```python
from build123d import *

# Parameters (mm, degrees)
F1_DEPTH = 9
F2_DEPTH = 2


with BuildPart() as f1:
    # F0 (on Top) → F1 (new body)
    with BuildSketch(Plane.XY):
        with BuildLine():
            ThreePointArc((3.4640958416, -2), (3.863698102, -1.0352762805), (3.999995, 0))
            ThreePointArc((3.999995, 0), (3.863698102, 1.0352762805), (3.4640958416, 2))
            Line((3.4640958416, 2), (-3.4640958416, 2))
            ThreePointArc((-3.4640958416, 2), (-3.999995, 0), (-3.4640958416, -2))
            Line((-3.4640958416, -2), (3.4640958416, -2))
        make_face()
        with BuildLine():
            Line((-3.4640958416, 2), (3.4640958416, 2))
            ThreePointArc((3.4640958416, 2), (0, 3.999995), (-3.4640958416, 2))
        make_face()
        with BuildLine():
            ThreePointArc((-3.4640958416, -2), (0, -3.999995), (3.4640958416, -2))
            Line((3.4640958416, -2), (-3.4640958416, -2))
        make_face()
    extrude(amount=F1_DEPTH)

    # F0 (on Top) → F2 (join)
    with BuildSketch(Plane.XY):
        with BuildLine():
            ThreePointArc((3.4640958416, -2), (3.863698102, -1.0352762805), (3.999995, 0))
            ThreePointArc((3.999995, 0), (3.863698102, 1.0352762805), (3.4640958416, 2))
            Line((3.4640958416, 2), (-3.4640958416, 2))
            ThreePointArc((-3.4640958416, 2), (-3.999995, 0), (-3.4640958416, -2))
            Line((-3.4640958416, -2), (3.4640958416, -2))
        make_face()
        with BuildLine():
            ThreePointArc((3.4640958416, 2), (3.863698102, 1.0352762805), (3.999995, 0))
            ThreePointArc((3.999995, 0), (3.863698102, -1.0352762805), (3.4640958416, -2))
            Line((3.4640958416, -2), (8, -2))
            Line((8, -2), (8, 2))
            Line((8, 2), (3.4640958416, 2))
        make_face()
        with BuildLine():
            Line((-3.4640958416, 2), (3.4640958416, 2))
            ThreePointArc((3.4640958416, 2), (0, 3.999995), (-3.4640958416, 2))
        make_face()
        with BuildLine():
            ThreePointArc((-3.4640958416, -2), (0, -3.999995), (3.4640958416, -2))
            Line((3.4640958416, -2), (-3.4640958416, -2))
        make_face()
        with BuildLine():
            ThreePointArc((-3.4640958416, -2), (-3.999995, 0), (-3.4640958416, 2))
            Line((-3.4640958416, 2), (-8, 2))
            Line((-8, 2), (-8, -2))
            Line((-8, -2), (-3.4640958416, -2))
        make_face()
    extrude(amount=F2_DEPTH)


solid = f1.part
```
Model file for the job. Use its own axes, mm. A direction names the side the tool comes from. Coordinates: 2 decimals unless noted, no trailing zeros. Order: outer loops, then holes, each group sorted by start corner. A loop starts at its lowest first (then second) coordinate and runs counter-clockwise, first axis right, second up. Notation, with made-up numbers: (56.25, 41.25) -> (80.25, 41.25) arc R21 ccw to (80.25, 80.25) -> close; hole circle Ø9 at (72, 58.5). An arc over 180 degrees is marked (long way). Answer as a JSON object with one key per item and string values. Group by question number.
1) Drill centre lines: L1, parallel to X at y = -2, z = 6.75; L2, parallel to Z at x = -4, y = -0.5; L3, parallel to Y at x = -2.75, z = 2.25. Where is each one in solid material? Low to high.
2) Cut at A-A, the plane z = 1. Write the cut outline in (x, y).
3) Cut at B-B, the plane y = 0.25. Write the cut outline in (x, z), then the cut area to 3 significant figures.
4) Which spindle directions (+Z, -Z, +X, -X, +Y, -Y) get a long thin tool onto all of the face, cutting with end or side? Do faces 1 (the face through (-6, 2, 1)), 2 (the face through (6, -2, 1)), 3 (the face through (6, 2, 1)), 4 (the face through (8, 0, 1)). Say none if no direction does.
5) Pull direction Z, two halves, no side cores. Call faces 5 (the face through (6, 0, 2)), 6 (the face through (-6, -2, 1)), 7 (the face through (0, 0, 0)): +Z half, -Z half, draft (parallel to the pull), parting line (faces both ways), or undercut.
6) Cut at C-C, the plane x = 5.5. Write the cut outline in (y, z).
7) Flat gauge pins, fed straight in: pin 1 (1 mm diameter, centred on x = -5, z = 0.5, fed in from -Y); pin 2 (2 mm diameter, centred on x = 7, z = 1.5, fed in from +Y); pin 3 (3 mm diameter, centred on y = 1, z = 6.5, fed in from -X); pin 4 (2 mm diameter, centred on x = -1, z = 6.5, fed in from +Y). Where does each tip first touch, or does it go through?
8) Cut at D-D, the plane z = 5.75. Write the cut outline in (x, y), then the cut area to 3 significant figures.
Check values:
{
 "1": {"L1": "x = -3.46 to 3.46", "L2": "z = 0 to 2", "L3": "y = -2.9 to 2.9"},
 "2": {"outline": "(-8, -2) -> (-3.46, -2) arc R4 ccw to (3.46, -2) -> (8, -2) -> (8, 2) -> (3.46, 2) arc R4 ccw to (-3.46, 2) -> (-8, 2) -> close"},
 "3": {"outline": "(-8, 0) -> (8, 0) -> (8, 2) -> (3.99, 2) -> (3.99, 9) -> (-3.99, 9) -> (-3.99, 2) -> (-8, 2) -> close", "area": "87.9 mm²"},
 "4": {"face 1": "+Z, -Z, -X, +Y", "face 2": "+Z, -Z, +X, -Y", "face 3": "+Z, -Z, +X, +Y", "face 4": "+Z, -Z, +X, +Y, -Y"},
 "5": {"face 5": "+Z half", "face 6": "draft", "face 7": "-Z half"},
 "6": {"outline": "(-2, 0) -> (2, 0) -> (2, 2) -> (-2, 2) -> close"},
 "7": {"pin 1": "stops at y = -2", "pin 2": "stops at y = 2", "pin 3": "stops at x = -4", "pin 4": "stops at y = 4"},
 "8": {"outline": "circle Ø8 at (0, 0)", "area": "50.3 mm²"}
}
